```python
from build123d import *

# Parameters (mm, degrees)
SM_BASE_FLANGE_1_DEPTH   = 550
SKETCH_6_W               = 3
SKETCH_6_H               = 71
CUT_EXTRUDE_1_DEPTH      = 681.413293521
SKETCH_7_W               = 3
SKETCH_7_H               = 69
SM_BASE_FLANGE_1_2_DEPTH = 1.5
SKETCH_10_R              = 3.5
CUT_EXTRUDE_2_DEPTH      = 10
SKETCH_11_R              = 6
CUT_EXTRUDE_1853_DEPTH   = 10


# Sheet-metal steps are written as plain solids
with BuildPart() as part:
    # Sketch 1 → Sm Base Flange 1 (new, symmetric)
    with BuildSketch(Plane.XY):
        with BuildLine():
            Line((-398.5, -20), (-398.5, -1.5))
            ThreePointArc((-398.5, -1.5), (-398.060660172, -0.439339828), (-397, 0))
            Line((-397, 0), (397, 0))
            ThreePointArc((397, 0), (398.060660172, -0.439339828), (398.5, -1.5))
            Line((398.5, -1.5), (398.5, -20))
            Line((398.5, -20), (400, -20))
            Line((400, -20), (400, -1.5))
            ThreePointArc((400, -1.5), (399.121320344, 0.621320344), (397, 1.5))
            Line((397, 1.5), (-397, 1.5))
            ThreePointArc((-397, 1.5), (-399.121320344, 0.621320344), (-400, -1.5))
            Line((-400, -1.5), (-400, -20))
            Line((-400, -20), (-398.5, -20))
        make_face()
    extrude(amount=SM_BASE_FLANGE_1_DEPTH, both=True)

    # Эскиз6 → Вырез-Вытянуть1 (cut, through all)
    with BuildSketch(Plane(origin=(0, 1.5, 0), x_dir=(1, 0, 0), z_dir=(0, 1, 0))):
        with Locations((398.5, -514.5)):
            Rectangle(SKETCH_6_W, SKETCH_6_H)
        with Locations((398.5, 514.5)):
            Rectangle(SKETCH_6_W, SKETCH_6_H)
        with Locations((-398.5, 514.5)):
            Rectangle(SKETCH_6_W, SKETCH_6_H)
        with Locations((-398.5, -514.5)):
            Rectangle(SKETCH_6_W, SKETCH_6_H)
    extrude(amount=-CUT_EXTRUDE_1_DEPTH, mode=Mode.SUBTRACT)

    # Эскиз7 → Sm Base Flange 1 2 (add)
    with BuildSketch(Plane(origin=(0, 1.5, 0), x_dir=(1, 0, 0), z_dir=(0, 1, 0))):
        with Locations((398.5, -515.5)):
            Rectangle(SKETCH_7_W, SKETCH_7_H)
        with Locations((398.5, 515.5)):
            Rectangle(SKETCH_7_W, SKETCH_7_H)
        with Locations((-398.5, 515.5)):
            Rectangle(SKETCH_7_W, SKETCH_7_H)
        with Locations((-398.5, -515.5)):
            Rectangle(SKETCH_7_W, SKETCH_7_H)
    extrude(amount=-SM_BASE_FLANGE_1_2_DEPTH)

    # Эскиз10 → Вырез-Вытянуть2 (cut)
    with BuildSketch(Plane(origin=(0, 1.5, 0), x_dir=(1, 0, 0), z_dir=(0, 1, 0))):
        with Locations(Location((365, -516, 0), (0, 0, 270))):
            Circle(SKETCH_10_R)
        with Locations(Location((365, 516, 0), (0, 0, 90))):
            Circle(SKETCH_10_R)
        with Locations(Location((-365, 516, 0), (0, 0, 270))):
            Circle(SKETCH_10_R)
        with Locations(Location((-365, -516, 0), (0, 0, 90))):
            Circle(SKETCH_10_R)
    extrude(amount=-CUT_EXTRUDE_2_DEPTH, mode=Mode.SUBTRACT)

    # Эскиз11 → Cut-Extrude 1853 (cut)
    with BuildSketch(Plane(origin=(0, 1.5, 0), x_dir=(1, 0, 0), z_dir=(0, 1, 0))):
        with Locations(Location((161.75, -528, 0), (0, 0, 270))):
            Circle(SKETCH_11_R)
        with Locations(Location((48.25, -528, 0), (0, 0, 270))):
            Circle(SKETCH_11_R)
        with Locations(Location((48.25, 528, 0), (0, 0, 90))):
            Circle(SKETCH_11_R)
        with Locations(Location((161.75, 528, 0), (0, 0, 90))):
            Circle(SKETCH_11_R)
        with Locations(Location((-161.75, 528, 0), (0, 0, 270))):
            Circle(SKETCH_11_R)
        with Locations(Location((-48.25, 528, 0), (0, 0, 270))):
            Circle(SKETCH_11_R)
        with Locations(Location((-48.25, -528, 0), (0, 0, 90))):
            Circle(SKETCH_11_R)
        with Locations(Location((-161.75, -528, 0), (0, 0, 90))):
            Circle(SKETCH_11_R)
    extrude(amount=-CUT_EXTRUDE_1853_DEPTH, mode=Mode.SUBTRACT)


solid = part.part
```
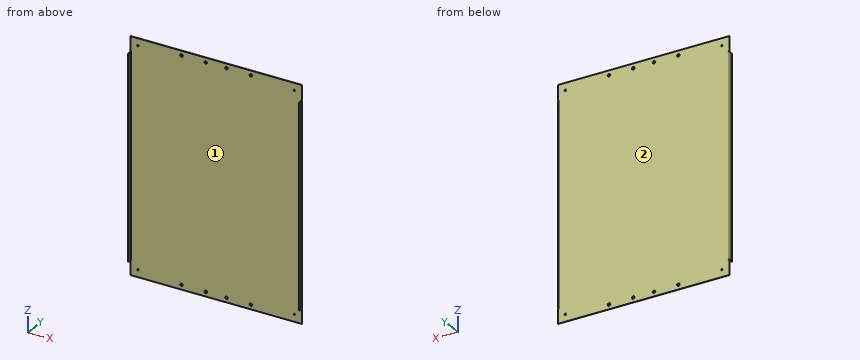
CAD build for the part. Positions are in the model's coordinates, mm. Face numbers are marked on the shaded views. Coordinates: 2 decimals unless noted, no trailing zeros. Write each loop counter-clockwise with the first axis right and the second up, starting at its lowest first coordinate (ties: lowest second). Pieces come first, ordered by that corner, then holes.
(1) Cut at B-B, the plane z = 1. List the corners of the cut face in (x, y), and give its area (3 significant figures).
(2) Cut at A-A, the plane y = -15.25. List the corners of the cut face in (x, z), and give its area (3 significant figures).
(3) Cut at C-C, the plane x = -286.5. List the corners of the cut face in (y, z).
(4) Two-plate mould, pull along X, no slides. Class the marked faces 1 and 2: +X half, -X half, draft (parallel to the pull), parting line (faces both ways), or undercut.
(5) Drill centre lines: probe 1 along X at (y, z) = (0.75, -528); probe 2 along X at (y, z) = (1.15, 516); probe 3 along X at (y, z) = (-5.5, 258.5). Where is each one in solid material? Low to high.
(6) Flat gauge pins, fed straight in: pin 1 (15.5 mm diameter, centred on x = -161.75, z = -528, fed in from -Y); pin 2 (9.5 mm diameter, centred on x = 48.25, z = -528, fed in from +Y); pin 3 (0.5 mm diameter, centred on y = 1, z = 480.5, fed in from +X). Where does each tip first touch, or does it go through?
Geometry says:
1. outline: (-400, -20) - (-398.5, -20) - (-398.5, -1.5) arc R1.5 cw to (-397, 0) - (397, 0) arc R1.5 cw to (398.5, -1.5) - (398.5, -20) - (400, -20) - (400, -1.5) arc R3 ccw to (397, 1.5) - (-397, 1.5) arc R3 ccw to (-400, -1.5) - close
1. area: 1,260 mm2
2. outline: (-400, -479) - (-398.5, -479) - (-398.5, 479) - (-400, 479) - close; (398.5, -479) - (400, -479) - (400, 479) - (398.5, 479) - close
2. area: 2,870 mm2
3. outline: (0, -550) - (1.5, -550) - (1.5, 550) - (0, 550) - close
4. face 1: undercut
4. face 2: draft
5. probe 1: x = -400 to -167.75, -155.75 to -54.25, -42.25 to 42.25, 54.25 to 155.75, 167.75 to 400
5. probe 2: x = -400 to -368.5, -361.5 to 361.5, 368.5 to 400
5. probe 3: x = -400 to -398.5, 398.5 to 400
6. pin 1: stops at y = 0
6. pin 2: passes through
6. pin 3: stops at x = 397
